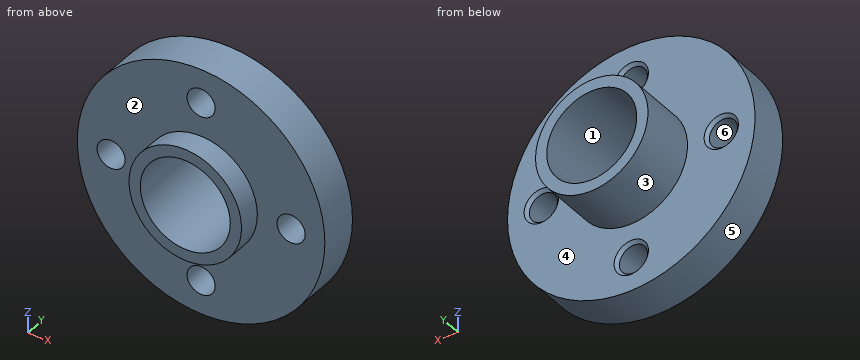
from build123d import *

# Parameters (mm, degrees)
SKETCH_1_R                   = 11
EXTRUDE_1_DEPTH              = 3.5
SKETCH_2_R                   = 5
EXTRUDE_2_DEPTH              = 5
EXTRUDE_2_DEPTH_BACK         = 5.5
SKETCH_3_R                   = 1.15
CUT_EXTRUDE_1_DEPTH          = 5
SKETCH_4_R                   = 4
CUT_EXTRUDE_2_DEPTH          = 11.5
HOLE_WIZARD_M3_1_D           = 2.5
HOLE_WIZARD_M3_1_DEPTH       = 8.5
HOLE_WIZARD_M3_1_CSINK_D     = 3.05
HOLE_WIZARD_M3_1_CSINK_ANGLE = 90
HOLE_WIZARD_M3_1_TIP         = 0.751075774


with BuildPart() as part:
    # 草图1 → 凸台-拉伸1 (new body)
    with BuildSketch(Plane(origin=(0, 0, 0), x_dir=(1, 0, 0), z_dir=(0, 1, 0))):
        Circle(SKETCH_1_R)
    extrude(amount=EXTRUDE_1_DEPTH)

    # 草图2 → 凸台-拉伸2 (add, two sides)
    with BuildSketch(Plane(origin=(0, 3.5, 0), x_dir=(1, 0, 0), z_dir=(0, 1, 0))) as extrude_2_sk:
        Circle(SKETCH_2_R)
    extrude(amount=EXTRUDE_2_DEPTH)
    extrude(extrude_2_sk.sketch, amount=-EXTRUDE_2_DEPTH_BACK)

    # 草图3 → 切除-拉伸1 (cut)
    with BuildSketch(Plane(origin=(0, 3.5, 0), x_dir=(1, 0, 0), z_dir=(0, 1, 0))):
        with Locations((0, 8)):
            Circle(SKETCH_3_R)
        with Locations((8, 0)):
            Circle(SKETCH_3_R)
        with Locations((0, -8)):
            Circle(SKETCH_3_R)
        with Locations((-8, 0)):
            Circle(SKETCH_3_R)
    extrude(amount=-CUT_EXTRUDE_1_DEPTH, mode=Mode.SUBTRACT)

    # 草图4 → 切除-拉伸2 (cut, through all)
    with BuildSketch(Plane(origin=(0, 8.5, 0), x_dir=(1, 0, 0), z_dir=(0, 1, 0))):
        Circle(SKETCH_4_R)
    extrude(amount=-CUT_EXTRUDE_2_DEPTH, mode=Mode.SUBTRACT)

    # M3 螺纹孔1
    with Locations(Plane(origin=(0, 3.5, 0), x_dir=(1, 0, 0), z_dir=(0, 1, 0))):
        with Locations((0, 8), (8, 0), (0, -8), (-8, 0)):
            CounterSinkHole(HOLE_WIZARD_M3_1_D / 2, HOLE_WIZARD_M3_1_CSINK_D / 2, depth=HOLE_WIZARD_M3_1_DEPTH, counter_sink_angle=HOLE_WIZARD_M3_1_CSINK_ANGLE)
            with Locations((0, 0, -(HOLE_WIZARD_M3_1_DEPTH + HOLE_WIZARD_M3_1_TIP / 2))):  # 118° drill point
                Cone(0, HOLE_WIZARD_M3_1_D / 2, HOLE_WIZARD_M3_1_TIP, mode=Mode.SUBTRACT)


solid = part.part
Build history of the part. All positions in model axes, mm. Face numbers are marked on the shaded views. A direction names the side the tool comes from. Give positions to 0.01 mm unless a question says otherwise; leave off trailing zeros. Write each loop counter-clockwise with the first axis right and the second up, starting at its lowest first coordinate (ties: lowest second). Pieces come first, ordered by that corner, then holes. Notation, with made-up numbers: (-5.75, 14) - (3.25, 14) arc R23 cw to (3.25, 23) - close; hole circle Ø4 at (6, -25.5). An arc over 180 degrees is marked (long way). Use one line per item in the form item = value. Start each with the question number.
1. Band-saw the part on A-A on x = 0. Write the cut outline in (y, z) (3 decimals).
2. Band-saw the part on D-D on x = -2.5. Write the cut outline in (y, z), plus the area to 3 significant figures.
3. Band-saw the part on B-B on z = 0. Write the cut outline in (x, y) (3 decimals), plus the area to 3 significant figures.
4. Probe line 1 (Z direction, x = 0, y = 2); line 2 (X direction, y = -0.5, z = 1.75); line 3 (Z direction, x = -8, y = 0.8). List the from-to ranges inside material, lowest first. Write a range as [from, to].
5. Drop flat-ended pins along their axis: pin 1 Ø1.5 at (x, z) = (-6.5, 2.5) entering from -Y; pin 2 Ø3 at (y, z) = (1, -0.5) entering from +X; pin 3 Ø5 at (x, z) = (-8, 6.5) entering from +Y. Give the stop position or say it passes through.
6. Two-plate mould, pull along Z, no slides. Class the marked faces 4, 5 and 6: released by +Z, released by -Z, zero draft, split by the parting line, or undercut.
7. Band-saw the part on C-C on z = -3.25. Write the cut outline in (x, y), plus the area to 3 significant figures.
8. 3-axis set-ups, long thin cutter, end or side, ignore diameter. For the marked faces 1, 2 and 3: which of +Z, -Z, +X, -X, +Y, -Y reach the whole face in a straight line?
Conclusion:
q1.outline = (-2, -5) - (0, -5) - (0, -6.75) - (3.225, -6.75) - (3.5, -6.475) - (3.5, -5) - (8.5, -5) - (8.5, -4) - (-2, -4) - close; (-2, 4) - (8.5, 4) - (8.5, 5) - (3.5, 5) - (3.5, 6.475) - (3.225, 6.75) - (0, 6.75) - (0, 5) - (-2, 5) - close; (0, -11) - (3.5, -11) - (3.5, -9.525) - (3.225, -9.25) - (0, -9.25) - close; (0, 9.25) - (3.225, 9.25) - (3.5, 9.525) - (3.5, 11) - (0, 11) - close
q2.outline = (-2, -4.33) - (0, -4.33) - (0, -10.71) - (3.5, -10.71) - (3.5, -4.33) - (8.5, -4.33) - (8.5, -3.12) - (-2, -3.12) - close; (-2, 3.12) - (8.5, 3.12) - (8.5, 4.33) - (3.5, 4.33) - (3.5, 10.71) - (0, 10.71) - (0, 4.33) - (-2, 4.33) - close
q2.area = 70.0 mm²
q3.outline = (-11, 0) - (-9.25, 0) - (-9.25, 3.225) - (-9.525, 3.5) - (-11, 3.5) - close; (-6.75, 0) - (-5, 0) - (-5, -2) - (-4, -2) - (-4, 8.5) - (-5, 8.5) - (-5, 3.5) - (-6.475, 3.5) - (-6.75, 3.225) - close; (4, -2) - (5, -2) - (5, 0) - (6.75, 0) - (6.75, 3.225) - (6.475, 3.5) - (5, 3.5) - (5, 8.5) - (4, 8.5) - close; (9.25, 0) - (11, 0) - (11, 3.5) - (9.525, 3.5) - (9.25, 3.225) - close
q3.area = 45.3 mm²
q4.line_1 = [-11, -9.25], [-6.75, -4], [4, 6.75], [9.25, 11]
q4.line_2 = [-4.68, -3.6], [3.6, 4.68]
q4.line_3 = [-7.55, -1.25], [1.25, 7.55]
q5.pin_1 = 0
q5.pin_2 = 11
q5.pin_3 = 3.5
q6.face_4 = zero draft
q6.face_5 = split by the parting line
q6.face_6 = undercut
q7.outline = (-10.51, 0) - (-3.8, 0) - (-3.8, -2) - (-2.33, -2) - (-2.33, 8.5) - (-3.8, 8.5) - (-3.8, 3.5) - (-10.51, 3.5) - close; (2.33, -2) - (3.8, -2) - (3.8, 0) - (10.51, 0) - (10.51, 3.5) - (3.8, 3.5) - (3.8, 8.5) - (2.33, 8.5) - close
q7.area = 77.8 mm²
q8.face_1 = +Y, -Y
q8.face_2 = -Y
q8.face_3 = +Y
